The listing builds one solid part. Answer for the finished solid, in the listing's coordinates (mm). Give positions to 0.01 mm unless a question says otherwise; leave off trailing zeros. Order: outer loops, then holes, each group sorted by start corner. A loop starts at its lowest first (then second) coordinate and runs counter-clockwise, first axis right, second up. Notation, with made-up numbers: (13.5, 12) - (31.5, 12) arc R12 ccw to (31.5, 24) - close; hole circle Ø11 at (69.5, 23). An arc over 180 degrees is marked (long way). Answer as a JSON object with one key per item and string values. Group by question number.
Q1. A cutting plane is placed at C-C, the plane x = 9. Give the vertices of the cut face in (y, z), and give its area (3 significant figures).
Q2. Given pin 1 (2 mm diameter, centred on y = 0, z = 0, fed in from +X); pin 2 (1 mm diameter, centred on x = -10, y = -2, fed in from +Z); pin 3 (3 mm diameter, centred on x = 11.5, y = 2, fed in from -Z), each flat-ended and moving along its own axis, determine where each tip first touches the part or whether it passes through.
Q3. A cutting plane is placed at A-A, the plane z = 0. Give the vertices of the cut face in (x, y).
Q4. The mould has two halves that part along Z. Classify faces 1 (the face through (-25, 1, 2)), 2 (the face through (-0.347, 1.617, 0.67)), 3 (the face through (0, -3, 0)): released by +Z, released by -Z, zero draft, split by the parting line, or undercut.
Q5. Consider line 1 (Z direction, x = 11, y = 0); line 2 (Z direction, x = 3.5, y = -1.2); line 3 (Y direction, x = 14, z = -1.6). Determine where each line is inside the solid, lowest interval first.
Autodesk Inventor part; units mm, degrees
ref_plane "YZ Plane" through (0, 0, 0) normal (1, 0, 0) x (0, 1, 0)
ref_plane "XZ Plane" through (0, 0, 0) normal (0, 1, 0) x (-1, 0, 0)
ref_plane "XY Plane" through (0, 0, 0) normal (0, 0, 1) x (1, 0, 0)
sketch "スケッチ1" plane through (0, 0, 0) normal (1, 0, 0) x (0, 1, 0)
  circle A0 centre (0, 0) radius 3
  circle A1 centre (0, 0) radius 1.75
  dimension "d0" = 6
  dimension "d6" = 3.5
extrude "押し出し1" add sketch "スケッチ1" along normal mid plane 50
chamfer "面取り1" distance 0.2 angle 45 4 edges at (25, -3, 0) (-25, -3, 0) (25, -1.75, 0) (-25, -1.75, 0)
properties part number "KNEE_DRIVER_SHAFT"
Reply:
{
 "1": {"outline": "circle Ø6 at (0, 0); hole circle Ø3.5 at (0, 0)", "area": "18.7 mm^2"},
 "2": {"pin 1": "passes through", "pin 2": "stops at z = 2.6", "pin 3": "stops at z = -2.96"},
 "3": {"outline": "(-25, -2.8) - (-24.8, -3) - (24.8, -3) - (25, -2.8) - (25, -1.95) - (24.8, -1.75) - (-24.8, -1.75) - (-25, -1.95) - close; (-25, 1.95) - (-24.8, 1.75) - (24.8, 1.75) - (25, 1.95) - (25, 2.8) - (24.8, 3) - (-24.8, 3) - (-25, 2.8) - close"},
 "4": {"face 1": "zero draft", "face 2": "undercut", "face 3": "split by the parting line"},
 "5": {"line 1": "z = -3 to -1.75, 1.75 to 3", "line 2": "z = -2.75 to -1.27, 1.27 to 2.75", "line 3": "y = -2.54 to -0.71, 0.71 to 2.54"}
}
